Geometry check sheet. Reference: drawing and pictorial views, mm from the part's lowest x, y, z. Coordinates: 2 decimals unless noted, no trailing zeros. Loops run counter-clockwise (first coordinate to the right, second up) from the corner with the lowest first, then second, coordinate; pieces in that order, holes last.
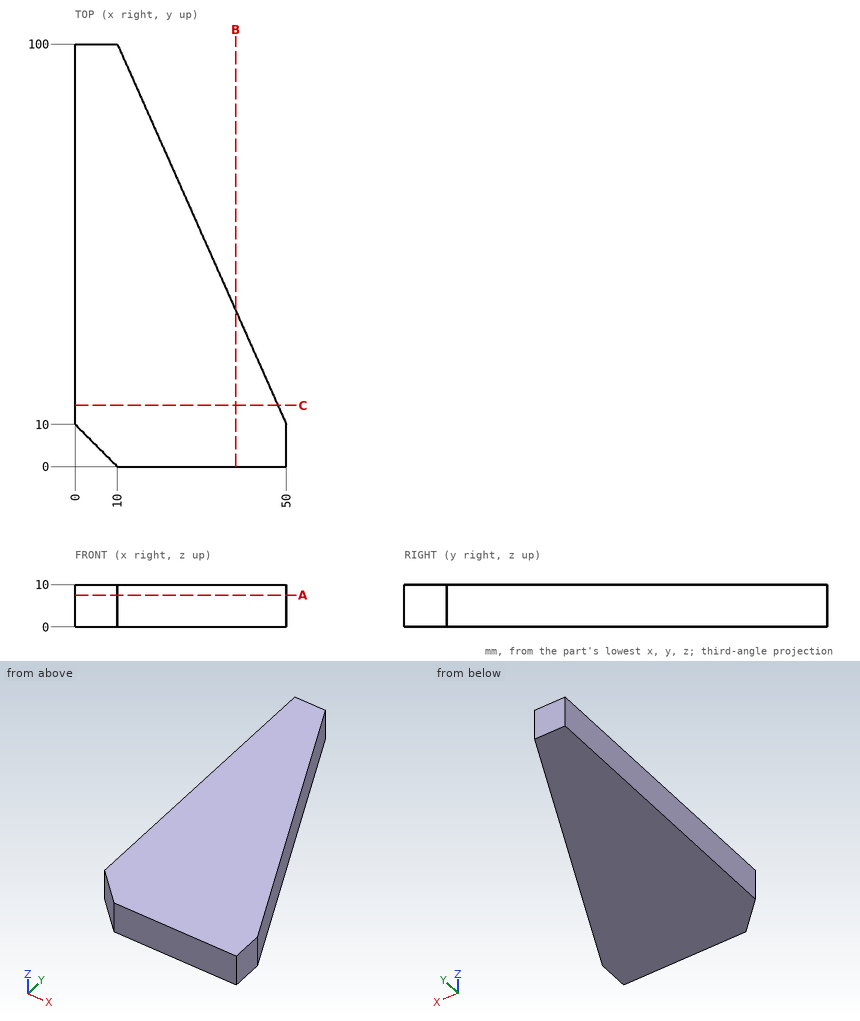
1) Section check C-C on y = 14.5. Record the cut outline in (x, z), and give its area (3 significant figures).
Data:
outline: (0, 0) - (48, 0) - (48, 10) - (0, 10) - close
area: 480 mm2
2) Section check A-A on z = 7.5. Record the cut outline in (x, y), and give its area (3 significant figures).
Data:
outline: (0, 10) - (10, 0) - (50, 0) - (50, 10) - (10, 100) - (0, 100) - close
area: 3,150 mm2
3) Material ranges on probe 1 along Y at (x, z) = (26.5, 7.5) (3 decimals); probe 2 along Y at (x, z) = (25, 6.25); probe 3 along X at (y, z) = (27.5, 6.75), recorded low to high.
Data:
probe 1: y = 0 to 62.875
probe 2: y = 0 to 66.25
probe 3: x = 0 to 42.22
4) Depth check by flat-ended pin: pin 1 (1.5 mm diameter, centred on x = 21.5, y = 20, fed in from -Z); pin 2 (1 mm diameter, centred on y = 53, z = 4.5, fed in from +X); pin 3 (5 mm diameter, centred on y = 17, z = 4, fed in from +X). Enter the tip coordinate at first touch or a pass-through.
Data:
pin 1: stops at z = 0
pin 2: stops at x = 31.11
pin 3: stops at x = 48
5) Section check B-B on x = 38. Record the cut outline in (y, z), and give its area (3 significant figures).
Data:
outline: (0, 0) - (37, 0) - (37, 10) - (0, 10) - close
area: 370 mm2
